Source: three-view drawing plus pictorial views. Frame: mm from the lowest corner of the part. A direction names the side the tool comes from. Give positions to 0.01 mm unless a question says otherwise; leave off trailing zeros. Loops run counter-clockwise (first coordinate to the right, second up) from the corner with the lowest first, then second, coordinate; pieces in that order, holes last. Notation, with made-up numbers: (71, 63.5) - (77, 63.5) arc R26 cw to (77, 90.5) - close; hole circle Ø5 at (-35, 86.5). An arc over 180 degrees is marked (long way). Answer as a JSON object with one key per item and string values.
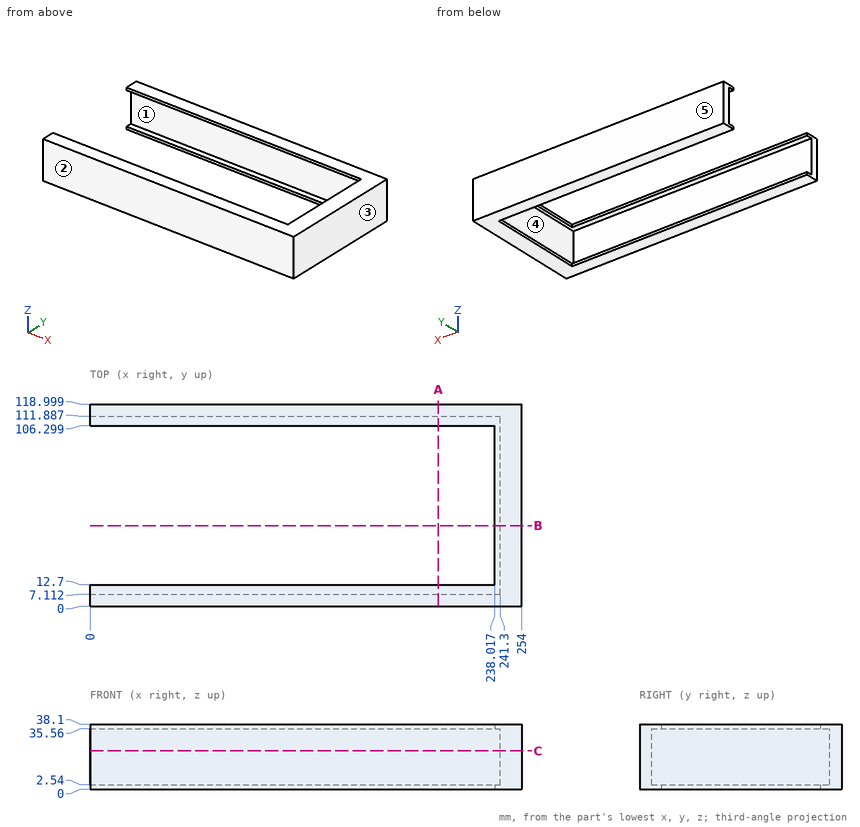
Item 1: Cut plane A-A (x = 205). Return loops of the section in (y, z).
Geometry check:
{"outline": "(0, 0) - (12.7, 0) - (12.7, 2.54) - (7.11, 2.54) - (7.11, 35.56) - (12.7, 35.56) - (12.7, 38.1) - (0, 38.1) - close; (106.3, 0) - (119, 0) - (119, 38.1) - (106.3, 38.1) - (106.3, 35.56) - (111.89, 35.56) - (111.89, 2.54) - (106.3, 2.54) - close"}
Item 2: Material intervals for line 1 (Y direction, x = 57, z = 21); line 2 (Y direction, x = 196, z = 36); line 3 (Z direction, x = 116, y = 110.5), sorted ascending. Write a range as [from, to].
Geometry check:
{"line 1": "y = [0, 7.11], [111.89, 119]", "line 2": "y = [0, 12.7], [106.3, 119]", "line 3": "z = [0, 2.54], [35.56, 38.1]"}
Item 3: Access query for the marked faces 4 and 5. Directions: +Z, -Z, +X, -X, +Y, -Y. A direction counts if a zero-diameter tool reaches every point of the face in a straight line with its end or side. Return the directions, or none.
Geometry check:
{"face 4": "-X", "face 5": "+Z, -Z, +X, -X, +Y"}
Item 4: Contact query for flat-ended pins moving along their axis: P1, Ø8, axis at y = 57.5, z = 4.5, coming from the -X side; P2, Ø5, axis at y = 88.5, z = 19.5, coming from the -X side. Output: stop coordinate, or through.
Geometry check:
{"P1": "stops at x = 238.02", "P2": "stops at x = 241.3"}
Item 5: Cut plane C-C (z = 22.5). Return loops of the section in (x, y), then the cut area to 3 significant figures.
Geometry check:
{"outline": "(0, 0) - (254, 0) - (254, 119) - (0, 119) - (0, 111.89) - (241.3, 111.89) - (241.3, 7.11) - (0, 7.11) - close", "area": "4,940 mm2"}
Item 6: Mould query, pull axis Y, two halves, no side actions, for the marked faces 1, 2 and 3. Classes: released by +Y, released by -Y, zero draft, split by the parting line, or undercut.
Geometry check:
{"face 1": "undercut", "face 2": "released by -Y", "face 3": "zero draft"}
Item 7: Cut plane B-B (y = 47.5). Return loops of the section in (x, z).
Geometry check:
{"outline": "(238.02, 0) - (254, 0) - (254, 38.1) - (238.02, 38.1) - (238.02, 35.56) - (241.3, 35.56) - (241.3, 2.54) - (238.02, 2.54) - close"}
